from build123d import *

# Parameters (mm, degrees)
BOSS_EXTRUDE1_DEPTH = 7.5
SKETCH3_R           = 2.1
CUT_EXTRUDE1_DEPTH  = 5


with BuildPart() as part:
    # Sketch1 → Boss-Extrude1 (new body)
    with BuildSketch(Plane.XY):
        Polygon((12.5, 75), (20, 75), (20, 60), (3.75, 60), (3.75, 0), (-3.75, 0), (-3.75, 60), (-20, 60), (-20, 75), (-12.5, 75), (-12.5, 67.5), (0, 67.5), (12.5, 67.5), align=None)
    extrude(amount=BOSS_EXTRUDE1_DEPTH)

    # Sketch3 → Cut-Extrude1 (cut)
    with BuildSketch(Plane(origin=(0, 75, 0), x_dir=(1, 0, 0), z_dir=(0, 1, 0))):
        with Locations(Location((-16.25, -3.75, 0), (0, 0, 270))):
            Circle(SKETCH3_R)
        with Locations(Location((16.25, -3.75, 0), (0, 0, 270))):
            Circle(SKETCH3_R)
    extrude(amount=-CUT_EXTRUDE1_DEPTH, mode=Mode.SUBTRACT)


solid = part.part
Model file for the job. Use its own axes, mm. A direction names the side the tool comes from. Coordinates: 2 decimals unless noted, no trailing zeros. Order: outer loops, then holes, each group sorted by start corner. A loop starts at its lowest first (then second) coordinate and runs counter-clockwise, first axis right, second up. Notation, with made-up numbers: (85.25, 65.5) -> (109.25, 65.5) arc R31 cw to (109.25, 94.5) -> close; hole circle Ø9 at (12.25, 17). An arc over 180 degrees is marked (long way). Return JSON: item names as keys, results as strings. Group by question number.
Item 1: Saw through at D-D on y = 24. Write the cut outline in (x, z).
Item 2: Flat gauge pins, fed straight in: P1, Ø1.5, axis at y = 46.5, z = 6, coming from the +X side; P2, Ø6, axis at x = 5, y = 22, coming from the +Z side; P3, Ø1.5, axis at y = 56, z = 2.5, coming from the -X side; P4, Ø1.3, axis at x = -15.5, z = 3.5, coming from the +Y side. Where does each tip first touch, or does it go through?
Item 3: Tool access for faces 1 (the flat face through (16, 70, 4)), 2 (the flat face through (12.5, 71, 4)), 3 (the flat face through (-3.75, 30, 4)): list every direction of +Z, -Z, +X, -X, +Y, -Y with a clear straight run to the whole face (end or side of a thin tool).
Item 4: Saw through at B-B on z = 3.75. Write the cut outline in (x, y).
Item 5: Saw through at C-C on x = 16.25. Write the cut outline in (y, z).
Item 6: Saw through at A-A on y = 69. Write the cut outline in (x, z).
Item 7: Wall check: line 1 along X through (y, z) = (72.65, 3.75); line 2 along Z through (x, y) = (-16, 74); line 3 along X through (y, z) = (4, 2). Give the ranges that are in metal, low to high. Write a range as [from, to].
Item 8: Pull direction Z, two halves, no side cores. Call faces 4 (the flat face through (0, 46, 0)), 5 (the cylindrical face through (-14.48, 72.54, 4.88)), 6 (the flat face through (18, 75, 2)): pulls with the +Z half, pulls with the -Z half, needs draft (parallel to the pull), parting line crosses it, or undercut.
Values found:
{
 "1": {"outline": "(-3.75, 0) -> (3.75, 0) -> (3.75, 7.5) -> (-3.75, 7.5) -> close"},
 "2": {"P1": "stops at x = 3.75", "P2": "stops at z = 7.5", "P3": "stops at x = -3.75", "P4": "stops at y = 70"},
 "3": {"face 1": "+Y", "face 2": "+Z, -Z, +Y", "face 3": "+Z, -Z, -X, -Y"},
 "4": {"outline": "(-20, 60) -> (-3.75, 60) -> (-3.75, 0) -> (3.75, 0) -> (3.75, 60) -> (20, 60) -> (20, 75) -> (18.35, 75) -> (18.35, 70) -> (14.15, 70) -> (14.15, 75) -> (12.5, 75) -> (12.5, 67.5) -> (-12.5, 67.5) -> (-12.5, 75) -> (-14.15, 75) -> (-14.15, 70) -> (-18.35, 70) -> (-18.35, 75) -> (-20, 75) -> close"},
 "5": {"outline": "(60, 0) -> (75, 0) -> (75, 1.65) -> (70, 1.65) -> (70, 5.85) -> (75, 5.85) -> (75, 7.5) -> (60, 7.5) -> close"},
 "6": {"outline": "(-20, 0) -> (-12.5, 0) -> (-12.5, 7.5) -> (-20, 7.5) -> close; (12.5, 0) -> (20, 0) -> (20, 7.5) -> (12.5, 7.5) -> close"},
 "7": {"line 1": "x = [-20, -18.35], [-14.15, -12.5], [12.5, 14.15], [18.35, 20]", "line 2": "z = [0, 1.66], [5.84, 7.5]", "line 3": "x = [-3.75, 3.75]"},
 "8": {"face 4": "pulls with the -Z half", "face 5": "undercut", "face 6": "needs draft"}
}
